Verification items for the finished model (mm, model axes). A direction names the side the tool comes from. Coordinates: 2 decimals unless noted, no trailing zeros. Order: outer loops, then holes, each group sorted by start corner. A loop starts at its lowest first (then second) coordinate and runs counter-clockwise, first axis right, second up. Notation, with made-up numbers: M 0.25,1.5 L 15.25,1.5 A30 cw 15.25,31.5 Z; hole C 87,78 d6. An arc over 180 degrees is marked long. Write item = value, one per line.
```python
from build123d import *

# Parameters (mm, degrees)
SKETCH1_R           = 13.85
BOSS_EXTRUDE1_DEPTH = 33.6
SKETCH2_R           = 3
BOSS_EXTRUDE2_DEPTH = 18
SKETCH4_R           = 1.215
SKETCH4_R_2         = 1.526666667
CUT_EXTRUDE1_DEPTH  = 8


with BuildPart() as part:
    # Sketch1 → Boss-Extrude1 (new body)
    with BuildSketch(Plane.XY):
        Circle(SKETCH1_R)
    extrude(amount=BOSS_EXTRUDE1_DEPTH)

    # Sketch2 → Boss-Extrude2 (add)
    with BuildSketch(Plane.XY.offset(33.6)):
        Circle(SKETCH2_R)
    extrude(amount=BOSS_EXTRUDE2_DEPTH)

    # Sketch4 → Cut-Extrude1 (cut)
    with BuildSketch(Plane(origin=(0, 0, 0), x_dir=(-1, 0, 0), z_dir=(0, 0, -1))):
        with Locations((-9.515, 0)):
            Circle(SKETCH4_R)
        with Locations((9.515, 0)):
            Circle(SKETCH4_R)
        with Locations((0, 7.593333333)):
            Circle(SKETCH4_R_2)
        with Locations((0, -7.593333333)):
            Circle(SKETCH4_R_2)
    extrude(amount=-CUT_EXTRUDE1_DEPTH, mode=Mode.SUBTRACT)


solid = part.part
```
Item 1: Release check for a two-part mould opening along X. For faces 1 (the cylindrical face through (-3, 0, 42)), 2 (the flat face through (0, -8, 8)), 3 (the flat face through (-0.2, 3.3, 33.6)) record: pulls with the +X half, pulls with the -X half, needs draft (parallel to the pull), parting line crosses it, or undercut.
Report:
face_1 = parting line crosses it
face_2 = undercut
face_3 = needs draft
Item 2: Tool access check on faces 4 (the flat face through (0, 0, 51.6)), 5 (the flat face through (10, 0, 8)). Record the directions out of +Z, -Z, +X, -X, +Y, -Y that give a thin tool (end or side, any length) a straight path to the whole face; none if there is none.
Report:
face_4 = +Z, +X, -X, +Y, -Y
face_5 = -Z
Item 3: Sectioned sample at B-B, the plane x = 0. Enter the section's corners in (y, z).
Report:
outline = M -13.85,0 L -9.12,0 L -9.12,8 L -6.07,8 L -6.07,0 L 6.07,0 L 6.07,8 L 9.12,8 L 9.12,0 L 13.85,0 L 13.85,33.6 L 3,33.6 L 3,51.6 L -3,51.6 L -3,33.6 L -13.85,33.6 Z
Item 4: Sectioned sample at C-C, the plane z = 44.5. Enter the section's corners in (x, y).
Report:
outline = C 0,0 d6
Item 5: Scan lines: L1, parallel to Y at x = 0, z = 6.25; L2, parallel to Z at x = 1.5, y = 11.25; L3, parallel to Y at x = -10.25, z = 5. Record each from-to range of solid material in increasing order. Write a range as from..to.
Report:
L1 = -13.85..-9.12, -6.07..6.07, 9.12..13.85
L2 = 0..33.6
L3 = -9.31..-0.97, 0.97..9.31
Item 6: Gauge pin test, flat ends, axial feed: pin 1 (1 mm diameter, centred on y = -1.5, z = 12, fed in from -X); pin 2 (2 mm diameter, centred on x = 9.515, y = 0, fed in from -Z); pin 3 (4 mm diameter, centred on x = 5.5, z = 38.5, fed in from +Y); pin 4 (8 mm diameter, centred on x = -9, z = 6.5, fed in from -Y). Record the tip position at first contact, or that the pin passes through.
Report:
pin_1 = -13.81
pin_2 = 8
pin_3 = through
pin_4 = -12.92
Item 7: Sectioned sample at D-D, the plane z = 11.5. Enter the section's corners in (x, y), then the cut area to 3 significant figures.
Report:
outline = C 0,0 d27.7
area = 603 mm^2
Item 8: Sectioned sample at A-A, the plane y = 0. Enter the section's corners in (x, z).
Report:
outline = M -13.85,0 L -10.73,0 L -10.73,8 L -8.3,8 L -8.3,0 L 8.3,0 L 8.3,8 L 10.73,8 L 10.73,0 L 13.85,0 L 13.85,33.6 L 3,33.6 L 3,51.6 L -3,51.6 L -3,33.6 L -13.85,33.6 Z
